from build123d import *

# Parameters (mm, degrees)
SKETCH_W     = 34.5
SKETCH_H     = 45
PAD_DEPTH    = 8.5
SKETCH001_W  = 4.2
SKETCH001_H  = 8.5
PAD001_DEPTH = 1.5
SKETCH002_W  = 4.2
SKETCH002_H  = 8.5
PAD002_DEPTH = 1.5


with BuildPart() as part:
    # Sketch → Pad (new body)
    with BuildSketch(Plane.XY):
        Rectangle(SKETCH_W, SKETCH_H)
    extrude(amount=PAD_DEPTH)

    # Sketch001 (on Face3 of Pad) → Pad001 (join)
    with BuildSketch(Plane.YZ.offset(17.25)):
        with Locations((0, 4.25)):
            Rectangle(SKETCH001_W, SKETCH001_H)
    extrude(amount=PAD001_DEPTH)

    # Sketch002 (on Face2 of Pad) → Pad002 (join)
    with BuildSketch(Plane.XZ.offset(22.5)):
        with Locations((0, 4.25)):
            Rectangle(SKETCH002_W, SKETCH002_H)
    extrude(amount=PAD002_DEPTH)


solid = part.part
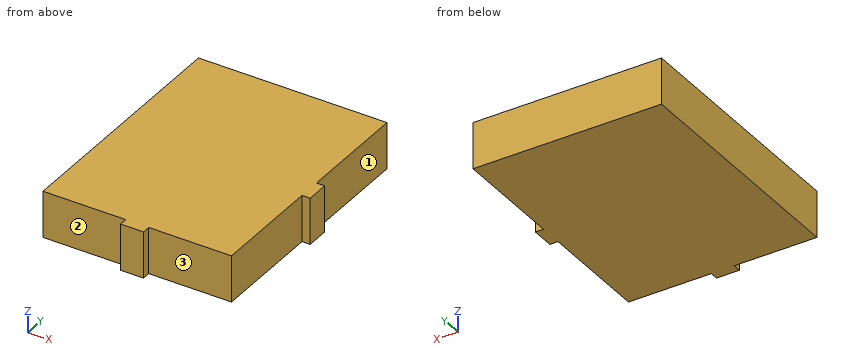
Can you work these out from the model? Positions are in its coordinate system, mm. Face numbers are marked on the shaded views. A direction names the side the tool comes from. Round coordinates to 2 decimals unless told otherwise and drop trailing zeros. Loops run counter-clockwise (first coordinate to the right, second up) from the corner with the lowest first, then second, coordinate; pieces in that order, holes last. Notation, with made-up numbers: (39.25, 27.5) - (60.25, 27.5) arc R11 ccw to (60.25, 33.5) - close; hole circle Ø9 at (-6, 30.25). An arc over 180 degrees is marked (long way). Write item = value, one per line. Start each with the question number.
(1) If I drill on probe 1 along X at (y, z) = (-11, 2); probe 2 along Y at (x, z) = (-11, 6.5), over which ranges is the centre line in solid material (lowest first)? Write a range as [from, to].
(2) For the marked faces 1, 2 and 3, which set-ups out of +Z, -Z, +X, -X, +Y, -Y let a thin tool reach every point of the face, with its end or its side?
(3) For P1, Ø1.6, axis at x = 18, z = 2.5, coming from the +Y side; P2, Ø1.2, axis at x = 17.5, z = 2.5, coming from the -Y side; P3, Ø1.6, axis at y = -23.5, z = 4, coming from the +X side; P4, Ø2.5, axis at y = -13, z = 2.5, coming from the +X side, each with a flat end and sliding along its axis, tell me the tip position at first contact or that it passes through.
(4) If we section it at C-C (y = -13): Please give me the cut outline in (x, z).
(5) If we section it at A-A (z = 2): Please give me the cut outline in (x, y).
(6) If we section it at B-B (x = 8.5): Please give me the cut outline in (y, z), and give its area (4 significant figures).
Ans:
q1.probe_1 = [-17.25, 17.25]
q1.probe_2 = [-22.5, 22.5]
q2.face_1 = +Z, -Z, +X, +Y
q2.face_2 = +Z, -Z, -X, -Y
q2.face_3 = +Z, -Z, +X, -Y
q3.P1 = 22.5
q3.P2 = -22.5
q3.P3 = 2.1
q3.P4 = 17.25
q4.outline = (-17.25, 0) - (17.25, 0) - (17.25, 8.5) - (-17.25, 8.5) - close
q5.outline = (-17.25, -22.5) - (-2.1, -22.5) - (-2.1, -24) - (2.1, -24) - (2.1, -22.5) - (17.25, -22.5) - (17.25, -2.1) - (18.75, -2.1) - (18.75, 2.1) - (17.25, 2.1) - (17.25, 22.5) - (-17.25, 22.5) - close
q6.outline = (-22.5, 0) - (22.5, 0) - (22.5, 8.5) - (-22.5, 8.5) - close
q6.area = 382.5 mm²
